Here's how the part is built. I have some questions about the finished solid (model axes, mm). A direction names the side the tool comes from. Round coordinates to 2 decimals unless told otherwise and drop trailing zeros. Order: outer loops, then holes, each group sorted by start corner. A loop starts at its lowest first (then second) coordinate and runs counter-clockwise, first axis right, second up. Notation, with made-up numbers: M 2.5,82 L 34.5,82 A27 cw 34.5,120 Z; hole C 38.25,24 d8. An arc over 180 degrees is marked long. Use one line per item in the form item = value. Start each with the question number.
```python
from build123d import *

# Parameters (mm, degrees)
SKETCH1_R           = 19.0875
SKETCH1_R_2         = 17.5
BOSS_EXTRUDE1_DEPTH = 50
SKETCH2_R           = 17.5
SKETCH2_R_2         = 6
BOSS_EXTRUDE2_DEPTH = 5
SKETCH3_R           = 17.5
SKETCH3_R_2         = 9
BOSS_EXTRUDE3_DEPTH = 1
SKETCH4_R           = 17.5
SKETCH4_R_2         = 10
BOSS_EXTRUDE4_DEPTH = 12
SKETCH7_W           = 2.75
SKETCH7_H           = 19.0875


with BuildPart() as part:
    # Sketch1 → Boss-Extrude1 (new body)
    with BuildSketch(Plane.XY):
        Circle(SKETCH1_R)
        Circle(SKETCH1_R_2, mode=Mode.SUBTRACT)
    extrude(amount=BOSS_EXTRUDE1_DEPTH)

    # Sketch2 → Boss-Extrude2 (add)
    with BuildSketch(Plane(origin=(0, 0, 0), x_dir=(-1, 0, 0), z_dir=(0, 0, -1))):
        Circle(SKETCH2_R)
        Circle(SKETCH2_R_2, mode=Mode.SUBTRACT)
    extrude(amount=-BOSS_EXTRUDE2_DEPTH)

    # Sketch3 → Boss-Extrude3 (add)
    with BuildSketch(Plane.XY.offset(5)):
        Circle(SKETCH3_R)
        Circle(SKETCH3_R_2, mode=Mode.SUBTRACT)
    extrude(amount=BOSS_EXTRUDE3_DEPTH)

    # Sketch4 → Boss-Extrude4 (add)
    with BuildSketch(Plane.XY.offset(6)):
        Circle(SKETCH4_R)
        Circle(SKETCH4_R_2, mode=Mode.SUBTRACT)
    extrude(amount=BOSS_EXTRUDE4_DEPTH)

    # Sketch7 → M5 Clearance Hole1 (revolve, cut)
    with BuildSketch(Plane(origin=(0, 0, 39.120000392), x_dir=(0, 0, -1), z_dir=(1, 0, 0))):
        with Locations((1.375, 9.54375)):
            Rectangle(SKETCH7_W, SKETCH7_H)
    m5_clearance_hole1 = revolve(axis=Axis((0, -6.35, 39.120000392), (0, 1, 0)), mode=Mode.SUBTRACT)

    # Mirror1: M5 Clearance Hole1 across plane
    add(m5_clearance_hole1.mirror(Plane.ZX), mode=Mode.SUBTRACT)


solid = part.part
```
1) If we section it at A-A on x = 0: Write out the boundary of the cut face in (y, z).
2) Will these pins go through, and if not, where does the flat tip stop? pin 1 Ø4.5 at (x, z) = (0, 39.12) entering from -Y; pin 2 Ø17.5 at (x, y) = (3, -5.5) entering from +Z; pin 3 Ø12 at (x, z) = (13.5, 35.5) entering from +Y; pin 4 Ø14.5 at (x, y) = (0, 0) entering from +Z.
3) If we section it at B-B on y = 0: Write out the boundary of the cut face in (x, z).
4) On a 3-axis mill with a long thin cutter (end or side, diameter ignored), from which of +Z, -Z, +X, -X, +Y, -Y can I reach the whole of each face in a straight line? I mean faces 4 (the cylindrical face through (1.1, -18.2, 36.6)), 5 (the flat face through (8, -8, 18)). Say none if no direction works.
5) If we section it at C-C on z = 37.5: Write out the boundary of the cut face in (x, y) (1 decimal).
6) If I drill on line 1 (Z direction, x = 0, y = 18.35); line 2 (Y direction, x = 0, z = 28); line 3 (X direction, y = 1, z = 5.5), over which ranges is the centre line in solid material (lowest first)?
7) If we section it at D-D on z = 43: Write out the boundary of the cut face in (x, y) (1 decimal).
8) If we mould it in two halves opening along Y, with no side actions, what happens to faces 1 (the flat face through (17, -6, 50)), 2 (the cylindrical face through (-2.485, 18.925, 24.65)), 3 (the cylindrical face through (6, 0, 2))? For each: +Y half, -Y half, draft (parallel to the pull), parting line (faces both ways), or undercut.
Completed:
q1.outline = M -19.09,0 L -6,0 L -6,5 L -9,5 L -9,6 L -10,6 L -10,18 L -17.5,18 L -17.5,36.37 L -19.09,36.37 Z; M -19.09,41.87 L -17.5,41.87 L -17.5,50 L -19.09,50 Z; M 6,0 L 19.09,0 L 19.09,36.37 L 17.5,36.37 L 17.5,18 L 10,18 L 10,6 L 9,6 L 9,5 L 6,5 Z; M 17.5,41.87 L 19.09,41.87 L 19.09,50 L 17.5,50 Z
q2.pin_1 = through
q2.pin_2 = 18
q2.pin_3 = 17.55
q2.pin_4 = 5
q3.outline = M -19.09,0 L -6,0 L -6,5 L -9,5 L -9,6 L -10,6 L -10,18 L -17.5,18 L -17.5,50 L -19.09,50 Z; M 6,0 L 19.09,0 L 19.09,50 L 17.5,50 L 17.5,18 L 10,18 L 10,6 L 9,6 L 9,5 L 6,5 Z
q4.face_4 = +Y, -Y
q4.face_5 = +Z
q5.outline = M -2.2,-19 L -2.2,-17.4 A17.5 cw -2.2,17.4 L -2.2,19 A19.1 ccw Z; M 2.2,-19 A19.1 ccw 2.2,19 L 2.2,17.4 A17.5 cw 2.2,-17.4 Z
q6.line_1 = 0 to 36.37, 41.87 to 50
q6.line_2 = -19.09 to -17.5, 17.5 to 19.09
q6.line_3 = -19.06 to -8.94, 8.94 to 19.06
q7.outline = C 0,0 d38.2; hole C 0,0 d35
q8.face_1 = draft
q8.face_2 = parting line
q8.face_3 = undercut
